Could you check a few things on this model? Use its own coordinates, in mm. Face numbers are marked on the shaded views. A direction names the side the tool comes from. Round coordinates to 2 decimals unless told otherwise and drop trailing zeros. Loops run counter-clockwise (first coordinate to the right, second up) from the corner with the lowest first, then second, coordinate; pieces in that order, holes last. Notation, with made-up numbers: (68, 16) -> (118, 16) arc R10 ccw to (118, 21) -> close; hole circle Ø7 at (38, 57.5). An arc over 180 degrees is marked (long way). Put each result on its own line as item: value. Start each with the question number.
1. Imagine slicing it at A-A, the plane x = -21.5. Please give me the cut outline in (y, z), and give its area (3 significant figures).
2. I'm going to push flat-ended pins straight in: P1, Ø2.5, axis at y = 4, z = 32.5, coming from the -X side; P2, Ø3, axis at x = 2, y = 2.5, coming from the +Z side; P3, Ø10, axis at x = 13, z = 10, coming from the +Y side; P4, Ø10, axis at x = -15.5, z = -23.5, coming from the +Y side. Where does each tip first touch, or does it pass through?
3. I need wall thicknesses on line 1 (Y direction, x = -10, z = 21). Which ranges of the line are inside material? Lowest first, please. Write a range as [from, to].
4. Which directions (+Z, -Z, +X, -X, +Y, -Y) give clear straight access to the entire face, cutting with the end or side of a thin tool? Please do the marked faces 1 and 2.
5. Imagine slicing it at C-C, the plane z = 12. Please give me the cut outline in (x, y).
6. Imagine slicing it at D-D, the plane x = 18. Please give me the cut outline in (y, z).
7. Imagine slicing it at B-B, the plane y = 36.5. Please give me the cut outline in (x, z), and give its area (3 significant figures).
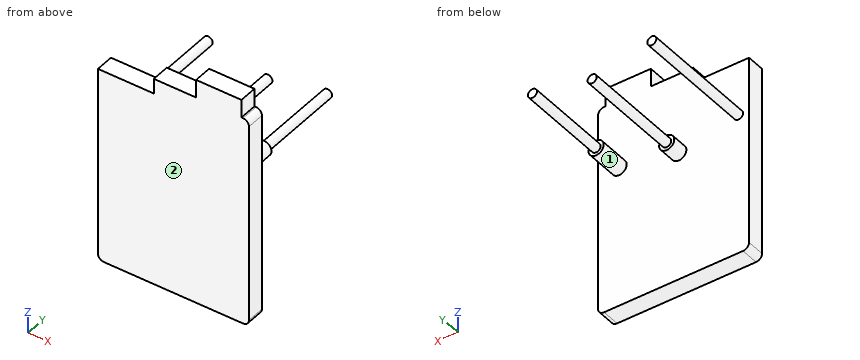
Autodesk Inventor part; units mm, degrees
ref_plane "YZ Plane" through (0, 0, 0) normal (1, 0, 0) x (0, 1, 0)
ref_plane "XZ Plane" through (0, 0, 0) normal (0, 1, 0) x (-1, 0, 0)
ref_plane "XY Plane" through (0, 0, 0) normal (0, 0, 1) x (1, 0, 0)
sketch "Sketch2" plane through (0, 0, 0) normal (0, 1, 0) x (-1, 0, 0)
  line L0 (25, -35) -> (-25, -35)
  line L1 (-25, -35) -> (-25, 35)
  line L2 (25, 30) -> (25, -35)
  line L3 (25, -35) -> (-25, 35) construction
  line L4 (-25, -35) -> (25, 35) construction
  line L5 (12, 35) -> (-3, 35)
  line L6 (6.5, 35) -> (12, 35)
  line L7 (-3, 35) -> (-25, 35)
  line L8 (25, 35) -> (6.5, 35)
  line L9 (6.5, 35) -> (6.5, 30)
  line L10 (6.5, 30) -> (25, 30)
  line L11 (25, 30) -> (25, 35)
  line L12 (-22.5, 35) -> (-7.5, 35)
  line L13 (-7.5, 35) -> (-7.5, 41)
  line L14 (-7.5, 41) -> (-22.5, 41)
  line L15 (-22.5, 41) -> (-22.5, 35)
  point P0 (0, 0)
  point P1 (0, 0)
  point P2 (-7.5, 35)
  dimension "d0" = 50
  dimension "d1" = 70
  dimension "d16" = 18.5
  dimension "d17" = 5
  dimension "d58" = 2.5
  dimension "d59" = 15
  dimension "d60" = 6
extrude "Extrusion3" add sketch "Sketch2" along normal blind 6 contours L0 L1 L7 L5 L9 L10 L2 | L15 L14 L13 L7
fillet "Fillet1" radius 2 3 edges at (25, 3, -35) (-25, 3, -35) (25, 3, 35)
sketch "Sketch4" plane through (0, 6, 0) normal (0, 1, 0) x (1, 0, 0)
  circle A0 centre (-1.75, -8) radius 2.5
  line L0 (25, -33) -> (25, 33)
  circle A1 centre (-21.5, -12) radius 1.5
  line L1 (-25, 33) -> (-25, -30)
  circle A2 centre (18, -12) radius 2.5
  line L2 (-6.5, -35) -> (7.5, -35)
  point P0 (0, 0)
  dimension "d31" = 5
  dimension "d34" = 3
  dimension "d41" = 5
  dimension "d44" = 19.75
  dimension "d45" = 19.75
  dimension "d46" = 7
  dimension "d61" = 23
  dimension "d62" = 27
  dimension "d63" = 23
extrude "Extrusion5" add sketch "Sketch4" along normal blind 40 contours A1
extrude "Extrusion6" add sketch "Sketch4" along normal blind 5.6 contours A0
sketch "Sketch5" plane through (-1.75, 11.6, 8) normal (0, 1, 0) x (1, 0, 0)
  circle A0 centre (0, 0) radius 1.5
  point P0 (1.75, 8)
  dimension "d50" = 3
extrude "Extrusion7" add sketch "Sketch5" along normal blind 34.4
extrude "Extrusion8" add sketch "Sketch4" along normal blind 10.64 contours A2
sketch "Sketch6" plane through (18, 16.64, 12) normal (0, 1, 0) x (1, 0, 0)
  circle A0 centre (0, 0) radius 1.5
  point P0 (-18, 12)
  dimension "d55" = 3
extrude "Extrusion9" add sketch "Sketch6" along normal blind 29.36
properties part number "Pared_caja_reduccion"
Entries:
1. outline: (0, -35) -> (6, -35) -> (6, 10.5) -> (46, 10.5) -> (46, 13.5) -> (6, 13.5) -> (6, 30) -> (0, 30) -> close
1. area: 510 mm^2
2. P1: x = -6.5
2. P2: z = 35
2. P3: y = 46
2. P4: y = 6
3. line 1: [0, 6]
4. face 1: +Y
4. face 2: +Z, -Z, +X, -X, -Y
5. outline: (-25, 0) -> (25, 0) -> (25, 6) -> (20.5, 6) -> (20.5, 16.64) -> (19.5, 16.64) -> (19.5, 46) -> (16.5, 46) -> (16.5, 16.64) -> (15.5, 16.64) -> (15.5, 6) -> (-20, 6) -> (-20, 46) -> (-23, 46) -> (-23, 6) -> (-25, 6) -> close
6. outline: (0, -35) -> (6, -35) -> (6, 9.5) -> (16.64, 9.5) -> (16.64, 10.5) -> (46, 10.5) -> (46, 13.5) -> (16.64, 13.5) -> (16.64, 14.5) -> (6, 14.5) -> (6, 41) -> (0, 41) -> close
7. outline: circle Ø3 at (-21.5, 12); circle Ø3 at (-1.75, 8); circle Ø3 at (18, 12)
7. area: 21.2 mm^2
